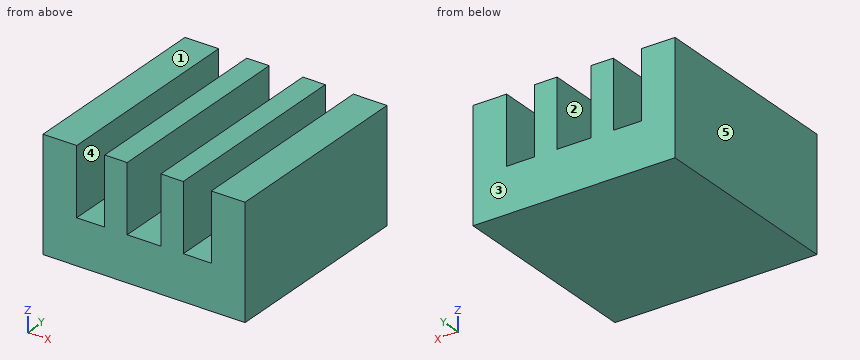
```python
from build123d import *

# Parameters (mm, degrees)
SKETCH_1_W          = 9
SKETCH_1_H          = 9
EXTRUDE_1_DEPTH     = 5
SKETCH_2_W          = 1.25
SKETCH_2_H          = 3
SKETCH_2_W_2        = 0.75
CUT_EXTRUDE_1_DEPTH = 10


with BuildPart() as part:
    # 草图1 → 凸台-拉伸1 (new body)
    with BuildSketch(Plane.XY):
        with Locations((4.5, 4.5)):
            Rectangle(SKETCH_1_W, SKETCH_1_H)
    extrude(amount=EXTRUDE_1_DEPTH)

    # 草图2 → 切除-拉伸1 (cut)
    with BuildSketch(Plane.XZ):
        with Locations((2.125, 3.5)):
            Rectangle(SKETCH_2_W, SKETCH_2_H)
        with Locations((4.125, 3.5)):
            Rectangle(SKETCH_2_W_2, SKETCH_2_H)
        with Locations((4.875, 3.5)):
            Rectangle(SKETCH_2_W_2, SKETCH_2_H)
        with Locations((6.875, 3.5)):
            Rectangle(SKETCH_2_W, SKETCH_2_H)
    extrude(amount=-CUT_EXTRUDE_1_DEPTH, mode=Mode.SUBTRACT)


solid = part.part
```
The listing builds one solid part. Answer for the finished solid, in the listing's coordinates (mm). Face numbers are marked on the shaded views. A direction names the side the tool comes from. Give positions to 0.01 mm unless a question says otherwise; leave off trailing zeros. Loops run counter-clockwise (first coordinate to the right, second up) from the corner with the lowest first, then second, coordinate; pieces in that order, holes last. Notation, with made-up numbers: (-13.5, 17) - (9.5, 17) arc R13 ccw to (9.5, 35) - close; hole circle Ø5 at (46, 15). An arc over 180 degrees is marked (long way). Return JSON: item names as keys, results as strings. Group by question number.
1. Find section C-C (x = 1.75). Write down the section's boundary in (y, z).
2. Determine the mould class of the marked faces 3, 4 and 5 for opening direction X: pulls with the +X half, pulls with the -X half, needs draft (parallel to the pull), parting line crosses it, or undercut.
3. Find section B-B (y = 3). Write down the section's boundary in (x, z), then the cut area to 3 significant figures.
4. Which of the six approach directions +Z, -Z, +X, -X, +Y, -Y give full straight-line access (tool end or side, diameter ignored) to the marked faces 1 and 2?
5. Straight lines are drawn through the part: line 1 (X direction, y = 6, z = 2.05); line 2 (Z direction, x = 4, y = 8.75). For each, find the intervals that lie inside material, in ascending order. Write a range as [from, to].
6. Find section A-A (z = 3.5). Write down the section's boundary in (x, y).
Verdict:
{
 "1": {"outline": "(0, 0) - (9, 0) - (9, 2) - (0, 2) - close"},
 "2": {"face 3": "needs draft", "face 4": "undercut", "face 5": "pulls with the -X half"},
 "3": {"outline": "(0, 0) - (9, 0) - (9, 5) - (7.5, 5) - (7.5, 2) - (6.25, 2) - (6.25, 5) - (5.25, 5) - (5.25, 2) - (3.75, 2) - (3.75, 5) - (2.75, 5) - (2.75, 2) - (1.5, 2) - (1.5, 5) - (0, 5) - close", "area": "33.0 mm^2"},
 "4": {"face 1": "+Z, +X, -X, +Y, -Y", "face 2": "+Z, +Y, -Y"},
 "5": {"line 1": "x = [0, 1.5], [2.75, 3.75], [5.25, 6.25], [7.5, 9]", "line 2": "z = [0, 2]"},
 "6": {"outline": "(0, 0) - (1.5, 0) - (1.5, 9) - (0, 9) - close; (2.75, 0) - (3.75, 0) - (3.75, 9) - (2.75, 9) - close; (5.25, 0) - (6.25, 0) - (6.25, 9) - (5.25, 9) - close; (7.5, 0) - (9, 0) - (9, 9) - (7.5, 9) - close"}
}
